from build123d import *

# Parameters (mm, degrees)
SKETCH1_W           = 218.44
SKETCH1_H           = 127
BOSS_EXTRUDE1_DEPTH = 63.5
SKETCH2_W           = 30
SKETCH2_H           = 15
BOSS_EXTRUDE2_DEPTH = 30
CUT_EXTRUDE1_REACH  = 162.35
FILLET1_R           = 5


with BuildPart() as part:
    # Sketch1 → Boss-Extrude1 (new body)
    with BuildSketch(Plane(origin=(0, 0, 0), x_dir=(1, 0, 0), z_dir=(0, 1, 0))):
        Rectangle(SKETCH1_W, SKETCH1_H)
    extrude(amount=BOSS_EXTRUDE1_DEPTH)

    # Sketch2 → Boss-Extrude2 (add)
    with BuildSketch(Plane(origin=(0, 63.5, 0), x_dir=(1, 0, 0), z_dir=(0, 1, 0))):
        Rectangle(SKETCH2_W, SKETCH2_H)
    extrude(amount=BOSS_EXTRUDE2_DEPTH)

    # Sketch3 → Cut-Extrude1 (cut, up to next)
    with BuildSketch(Plane(origin=(0, 0, -7.5), x_dir=(-1, 0, 0), z_dir=(0, 0, -1)), mode=Mode.PRIVATE) as cut_extrude1_sk1:
        with BuildLine():
            ThreePointArc((4.25, 83.5), (3.00520382, 86.50520382), (0, 87.75))
            Line((0, 87.75), (0, 79.25))
            ThreePointArc((0, 79.25), (3.00520382, 80.49479618), (4.25, 83.5))
        make_face()
    cut_extrude1_tool1 = extrude(cut_extrude1_sk1.sketch, amount=-CUT_EXTRUDE1_REACH, mode=Mode.PRIVATE) & part.part
    # Sketch3 → Cut-Extrude1 (cut, up to next)
    with BuildSketch(Plane(origin=(0, 0, -7.5), x_dir=(-1, 0, 0), z_dir=(0, 0, -1)), mode=Mode.PRIVATE) as cut_extrude1_sk2:
        with BuildLine():
            Line((0, 79.25), (0, 87.75))
            ThreePointArc((0, 87.75), (-4.25, 83.5), (0, 79.25))
        make_face()
    cut_extrude1_tool2 = extrude(cut_extrude1_sk2.sketch, amount=-CUT_EXTRUDE1_REACH, mode=Mode.PRIVATE) & part.part
    # Sketch3 → Cut-Extrude1 (cut, up to next)
    with BuildSketch(Plane(origin=(0, 0, -7.5), x_dir=(-1, 0, 0), z_dir=(0, 0, -1)), mode=Mode.PRIVATE) as cut_extrude1_sk3:
        with BuildLine():
            ThreePointArc((4.25, 83.5), (3.00520382, 86.50520382), (0, 87.75))
            Line((0, 87.75), (0, 79.25))
            ThreePointArc((0, 79.25), (3.00520382, 80.49479618), (4.25, 83.5))
        make_face()
    cut_extrude1_tool3 = extrude(cut_extrude1_sk3.sketch, amount=-CUT_EXTRUDE1_REACH, mode=Mode.PRIVATE) & part.part
    # Sketch3 → Cut-Extrude1 (cut, up to next)
    with BuildSketch(Plane(origin=(0, 0, -7.5), x_dir=(-1, 0, 0), z_dir=(0, 0, -1)), mode=Mode.PRIVATE) as cut_extrude1_sk4:
        with BuildLine():
            Line((0, 79.25), (0, 87.75))
            ThreePointArc((0, 87.75), (-4.25, 83.5), (0, 79.25))
        make_face()
    cut_extrude1_tool4 = extrude(cut_extrude1_sk4.sketch, amount=-CUT_EXTRUDE1_REACH, mode=Mode.PRIVATE) & part.part
    # Sketch3 → Cut-Extrude1 (cut, up to next)
    with BuildSketch(Plane(origin=(0, 0, -7.5), x_dir=(-1, 0, 0), z_dir=(0, 0, -1)), mode=Mode.PRIVATE) as cut_extrude1_sk5:
        with BuildLine():
            Line((15, 93.5), (0, 93.5))
            ThreePointArc((0, 93.5), (6.205203126, 91.341903734), (9.732121112, 85.799090834))
            Line((9.732121112, 85.799090834), (15, 63.5))
            Line((15, 63.5), (15, 93.5))
        make_face()
    cut_extrude1_tool5 = extrude(cut_extrude1_sk5.sketch, amount=-CUT_EXTRUDE1_REACH, mode=Mode.PRIVATE) & part.part
    # Sketch3 → Cut-Extrude1 (cut, up to next)
    with BuildSketch(Plane(origin=(0, 0, -7.5), x_dir=(-1, 0, 0), z_dir=(0, 0, -1)), mode=Mode.PRIVATE) as cut_extrude1_sk6:
        with BuildLine():
            ThreePointArc((-9.732121112, 85.799090834), (-6.205203126, 91.341903734), (0, 93.5))
            Line((0, 93.5), (-15, 93.5))
            Line((-15, 93.5), (-15, 63.5))
            Line((-15, 63.5), (-9.732121112, 85.799090834))
        make_face()
    cut_extrude1_tool6 = extrude(cut_extrude1_sk6.sketch, amount=-CUT_EXTRUDE1_REACH, mode=Mode.PRIVATE) & part.part
    add(cut_extrude1_tool1.solids().sort_by_distance((-1.803756, 83.5, -7.5))[0], mode=Mode.SUBTRACT)
    add(cut_extrude1_tool2.solids().sort_by_distance((1.803756, 83.5, -7.5))[0], mode=Mode.SUBTRACT)
    add(cut_extrude1_tool3.solids().sort_by_distance((-1.803756, 83.5, -7.5))[0], mode=Mode.SUBTRACT)
    add(cut_extrude1_tool4.solids().sort_by_distance((1.803756, 83.5, -7.5))[0], mode=Mode.SUBTRACT)
    add(cut_extrude1_tool5.solids().sort_by_distance((-12.015946, 84.357088, -7.5))[0], mode=Mode.SUBTRACT)
    add(cut_extrude1_tool6.solids().sort_by_distance((12.015946, 84.357088, -7.5))[0], mode=Mode.SUBTRACT)

    # Fillet1
    fillet1_edges = [part.edges().sort_by_distance(p)[0] for p in [
        (109.22, 63.5, 0),
        (0, 63.5, -63.5),
        (-109.22, 63.5, 0),
        (0, 0, -63.5),
        (109.22, 0, 0),
        (0, 0, 63.5),
        (-109.22, 0, 0),
        (0, 63.5, 63.5),
        (-109.22, 31.75, -63.5),
        (109.22, 31.75, -63.5),
        (109.22, 31.75, 63.5),
        (-109.22, 31.75, 63.5),
    ]]
    fillet(fillet1_edges, radius=FILLET1_R)


solid = part.part
Model file for the job. Use its own axes, mm. A direction names the side the tool comes from. Give positions to 0.01 mm unless a question says otherwise; leave off trailing zeros. Order: outer loops, then holes, each group sorted by start corner. A loop starts at its lowest first (then second) coordinate and runs counter-clockwise, first axis right, second up. Notation, with made-up numbers: M -25,66.25 L 34,66.25 A3 ccw 34,70.25 Z; hole C 81,41.25 d5. An arc over 180 degrees is marked long. Put each result on its own line as item: value. Start each with the question number.
(1) Band-saw the part on C-C on x = 95.5. Give the cut face in (y, z), then the cut area to 3 significant figures.
(2) Band-saw the part on A-A on z = -21.5. Give the cut face in (x, y), then the cut area to 3 significant figures.
(3) Tool access for faces 1 (the face through (107.72, 1.43, -0.82)), 2 (the face through (0, 75, -7.5)), 3 (the face through (0, 75, 7.5)): list every direction of +Z, -Z, +X, -X, +Y, -Y with a clear straight run to the whole face (end or side of a thin tool).
(4) Drill centre lines: L1, parallel to Y at x = 96, z = 17.5; L2, parallel to X at y = 87, z = 0.5. Where is each one in solid material? Low to high. Write a range as [from, to].
(5) Pin check, flat tips, straight feed: pin 1 Ø15 at (x, y) = (4, 73) entering from +Z; pin 2 Ø8 at (x, z) = (-86, 14.5) entering from +Y; pin 3 Ø5 at (y, z) = (77, 9) entering from +X. Stop position of each tip, or through.
(6) Band-saw the part on B-B on z = -1. Give the cut face in (x, y).
Results below:
1. outline: M 0,-58.5 A5 ccw 5,-63.5 L 58.5,-63.5 A5 ccw 63.5,-58.5 L 63.5,58.5 A5 ccw 58.5,63.5 L 5,63.5 A5 ccw 0,58.5 Z
1. area: 8,040 mm2
2. outline: M -109.22,5 A5 ccw -104.22,0 L 104.22,0 A5 ccw 109.22,5 L 109.22,58.5 A5 ccw 104.22,63.5 L -104.22,63.5 A5 ccw -109.22,58.5 Z
2. area: 13,800 mm2
3. face 1: +Z, -Z, +X, -Y
3. face 2: -Z, +X, -X, +Y
3. face 3: +Z, +X, -X, +Y
4. L1: y = [0, 63.5]
4. L2: x = [-9.37, -2.41], [2.41, 9.37]
5. pin 1: stops at z = 7.5
5. pin 2: stops at y = 63.5
5. pin 3: stops at x = 12.28
6. outline: M -109.22,5 A5 ccw -104.22,0 L 104.22,0 A5 ccw 109.22,5 L 109.22,58.5 A5 ccw 104.22,63.5 L 15,63.5 L 9.73,85.8 A10 ccw -9.73,85.8 L -15,63.5 L -104.22,63.5 A5 ccw -109.22,58.5 Z; hole C 0,83.5 d8.5
